from build123d import *

# Parameters (mm, degrees)
EXTRUDE1_DEPTH = 12


with BuildPart() as part:
    # Sketch1 → Revolve1 (revolve)
    with BuildSketch(Plane.XY, mode=Mode.PRIVATE) as revolve1_sk:
        with BuildLine():
            Line((0, 95.711947491), (-9, 95.711947491))
            Line((-9, 95.711947491), (-9, -1.288052509))
            ThreePointArc((-9, -1.288052509), (-9.585786438, -2.702266071), (-11, -3.288052509))
            Line((-11, -3.288052509), (-15, -3.288052509))
            Line((-15, -3.288052509), (-15, -45.288052509))
            Line((-15, -45.288052509), (-6, -45.288052509))
            Line((-6, -45.288052509), (-6, -13.288052509))
            Line((-6, -13.288052509), (0, -13.288052509))
            Line((0, -13.288052509), (0, 95.711947491))
        make_face()
    revolve(revolve1_sk.sketch.rotate(Axis((0, 0, 0), (0, 1, 0)), 270), axis=Axis((0, 0, 0), (0, 1, 0)))

    # Sketch2 → Extrude1 (add)
    with BuildSketch(Plane(origin=(0, 95.711947491, 0), x_dir=(-1, 0, 0), z_dir=(0, 1, 0))):
        Polygon((-6, 0), (0, -6), (6, 0), (0, 6), align=None)
    extrude(amount=EXTRUDE1_DEPTH)


solid = part.part
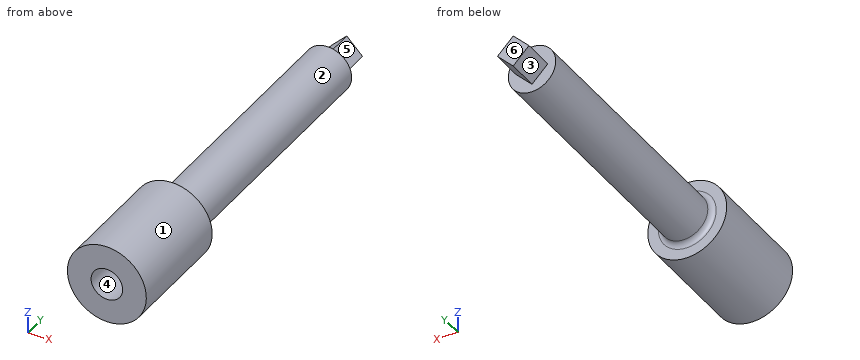
Source: CAD feature listing. Evaluate the final solid. Frame: model axes, mm. Face numbers are marked on the shaded views. A direction names the side the tool comes from. Give positions to 0.01 mm unless a question says otherwise; leave off trailing zeros. Write each loop counter-clockwise with the first axis right and the second up, starting at its lowest first coordinate (ties: lowest second). Pieces come first, ordered by that corner, then holes. Notation, with made-up numbers: M -15.5,19.25 L 23.5,19.25 A12 cw 23.5,39.25 Z; hole C 36,47.5 d10. An arc over 180 degrees is marked long. Return JSON: item names as keys, results as strings. Group by question number.
1) Draft query along Z for the marked faces 4, 5 and 6. Return one class per face: released by +Z, released by -Z, zero draft, split by the parting line, or undercut.
2) Cut plane B-B, the plane y = 78. Output: boundary loops of the cut face in (x, z), then the cut area to 3 significant figures.
3) Set-up query: the marked faces 1, 2 and 3. Return all of +Z, -Z, +X, -X, +Y, -Y with unobstructed straight access to the full face (end or side cutting, diameter ignored); none if empty.
4) Cut plane C-C, the plane z = -12.5. Output: boundary loops of the cut face in (x, y), then the cut area to 3 significant figures.
5) Cut plane A-A, the plane y = -17.5. Output: boundary loops of the cut face in (x, z), then the cut area to 3 significant figures.
6) First-contact query: pin 1 Ø4 at (y, z) = (71.5, -5) entering from -X; pin 2 Ø8 at (x, z) = (-12, -1.5) entering from +Y; pin 3 Ø3 at (x, y) = (-9.5, 18.5) entering from +Z. Flat tips, straight axial feed; report the tip coordinate or a pass-through.
7) Ray query, L1, parallel to X at y = -22, z = 0; L2, parallel to Y at x = -4.25, z = 3.75; L3, parallel to Z at x = 0.5, y = 88. Return the intervals inside material, ascending.
Data:
{
 "1": {"face 4": "undercut", "face 5": "released by +Z", "face 6": "zero draft"},
 "2": {"outline": "C 0,0 d18", "area": "254 mm²"},
 "3": {"face 1": "+Y, -Y", "face 2": "+Y", "face 3": "-Z, -X, +Y"},
 "4": {"outline": "M -8.29,-45.29 L 8.29,-45.29 L 8.29,-3.29 L -8.29,-3.29 Z", "area": "696 mm²"},
 "5": {"outline": "C 0,0 d30; hole C 0,0 d12", "area": "594 mm²"},
 "6": {"pin 1": "stops at x = -8.49", "pin 2": "stops at y = 95.71", "pin 3": "stops at z = 4.12"},
 "7": {"L1": "x = -15 to -6, 6 to 15", "L2": "y = -13.29 to 95.71", "L3": "z = -8.99 to 8.99"}
}
